from build123d import *

# Parameters (mm, degrees)
SKETCH1_R           = 2.75
SKETCH1_R_2         = 1.625
BOSS_EXTRUDE1_DEPTH = 5
SKETCH1_4_R         = 1.625
BOSS_EXTRUDE3_DEPTH = 13
CUT_EXTRUDE3_START  = 13
SKETCH1_6_R         = 1.6
CUT_EXTRUDE3_DEPTH  = 10


with BuildPart() as part:
    # Sketch1 → Boss-Extrude1 (new body)
    with BuildSketch(Plane(origin=(0, 0, 0), x_dir=(1, 0, 0), z_dir=(0, 1, 0))):
        Circle(SKETCH1_R)
        Circle(SKETCH1_R_2, mode=Mode.SUBTRACT)
    extrude(amount=BOSS_EXTRUDE1_DEPTH)

    # Sketch1<4> → Boss-Extrude3 (add)
    with BuildSketch(Plane(origin=(0, 0, 0), x_dir=(1, 0, 0), z_dir=(0, 1, 0))):
        Circle(SKETCH1_4_R)
    extrude(amount=BOSS_EXTRUDE3_DEPTH)

    # Sketch1<6> → Cut-Extrude3 (cut)
    with BuildSketch(Plane(origin=(0, 0, 0), x_dir=(1, 0, 0), z_dir=(0, 1, 0)).offset(CUT_EXTRUDE3_START)):
        with Locations((1.6, 0)):
            Circle(SKETCH1_6_R)
    extrude(amount=-CUT_EXTRUDE3_DEPTH, mode=Mode.SUBTRACT)


solid = part.part
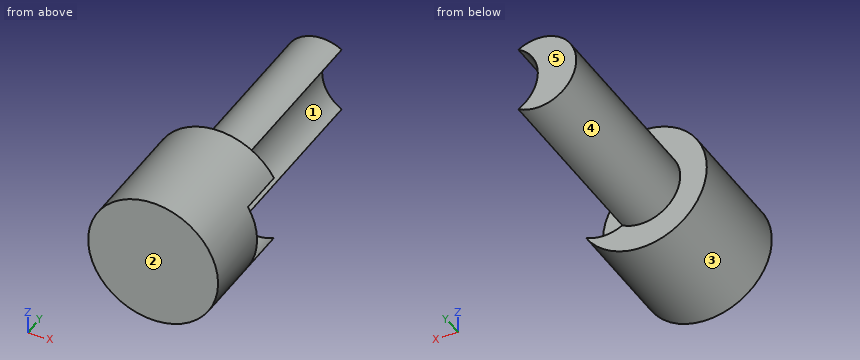
Input: part model. Units: mm. Frame: model coordinates. Face numbers are marked on the shaded views. A direction names the side the tool comes from. Give positions to 0.01 mm unless a question says otherwise; leave off trailing zeros. Loops run counter-clockwise (first coordinate to the right, second up) from the corner with the lowest first, then second, coordinate; pieces in that order, holes last. Notation, with made-up numbers: (22.5, 5) -> (49.5, 5) arc R13 cw to (49.5, 9) -> close; hole circle Ø5 at (21.25, -5.5). An arc over 180 degrees is marked (long way). Answer as a JSON object with one key per item and string values. Group by question number.
Item 1: Cut plane C-C, the plane x = 0.3. Return the cut outline in (y, z).
Item 2: Reachability of the marked faces 4 and 5 from +Z, -Z, +X, -X, +Y, -Y: full face, straight path, thin tool, end or side. Return the list, or none.
Item 3: Cut plane A-A, the plane x = 1.15. Return the cut outline in (y, z).
Item 4: Cut plane D-D, the plane y = 8. Return the cut outline in (x, z) (3 decimals).
Item 5: Pin query (flat end, axial travel): P1, Ø2, axis at x = 0.5, z = 0, coming from the +Y side; P2, Ø1.5, axis at x = 2, z = -2, coming from the +Y side; P3, Ø1, axis at x = -1, y = 8.5, coming from the -Z side. Return the tip coordinate at first contact, or that it passes through.
Item 6: Pull-direction query (Z, two-part tool) for the marked faces 1, 2 and 3; classes: released by +Z, released by -Z, zero draft, split by the parting line, or undercut.
Item 7: Line query: probe 1 along Y at (x, z) = (0.7, 0.55); probe 2 along X at (y, z) = (10.5, 0) (3 decimals); probe 3 along Y at (x, z) = (-2.25, 0.6). Output: solid intervals per line, ascending.
Item 8: Cut plane B-B, the plane z = 0. Return the cut outline in (x, y) (3 decimals).
Checks:
{
 "1": {"outline": "(0, -2.73) -> (5, -2.73) -> (5, -1.6) -> (13, -1.6) -> (13, -0.93) -> (3, -0.93) -> (3, 0.93) -> (13, 0.93) -> (13, 1.6) -> (5, 1.6) -> (5, 2.73) -> (0, 2.73) -> close"},
 "2": {"face 4": "+Y", "face 5": "+Z, -Z, +X, -X, +Y"},
 "3": {"outline": "(0, -2.5) -> (5, -2.5) -> (5, -1.54) -> (3, -1.54) -> (3, 1.54) -> (5, 1.54) -> (5, 2.5) -> (0, 2.5) -> close"},
 "4": {"outline": "(0.825, -1.4) arc R1.6 cw to (0.825, 1.4) arc R1.625 ccw (long way) to start"},
 "5": {"P1": "stops at y = 13", "P2": "stops at y = 5", "P3": "stops at z = -1.55"},
 "6": {"face 1": "undercut", "face 2": "zero draft", "face 3": "split by the parting line"},
 "7": {"probe 1": "y = 0 to 3", "probe 2": "x = -1.625 to 0", "probe 3": "y = 0 to 5"},
 "8": {"outline": "(-2.75, 0) -> (2.75, 0) -> (2.75, 3) -> (0, 3) -> (0, 13) -> (-1.625, 13) -> (-1.625, 5) -> (-2.75, 5) -> close"}
}
